Can you work these out from the model? Positions are in its coordinate system, mm. A direction names the side the tool comes from. Coordinates: 2 decimals unless noted, no trailing zeros. Loops run counter-clockwise (first coordinate to the right, second up) from the corner with the lowest first, then second, coordinate; pieces in that order, holes last. Notation, with made-up numbers: M 31.5,-39 L 59.5,-39 A27 cw 59.5,-3 Z; hole C 49.25,71 d3. An arc over 180 degrees is marked long. Answer as a JSON object with one key per item and string values. Group by question number.
Item 1: Suppose I cut it at D-D (x = 70). Write out the boundary of the cut face in (y, z).
Item 2: Suppose I cut it at C-C (z = 10). Count the separate pieces of the cut face and the enclosed holes in it, then the cut area to 3 significant figures.
Item 3: We'd pull the mould along Y, two halves only. Please class faces 1 (the flat face through (0, 27.7, 7.6)), 2 (the cylindrical face through (6.923, 48.226, 9.86)), 3 (the flat face through (27, 6, 7)): +Y half, -Y half, draft (parallel to the pull), parting line (faces both ways), or undercut.
Item 4: I'm going to push flat-ended pins straight in: pin 1 Ø10 at (y, z) = (30, 10) entering from +X; pin 2 Ø3.5 at (x, y) = (6, 50) entering from -Z; pin 3 Ø6 at (x, z) = (80.5, 10.5) entering from +Y; pin 4 Ø10 at (x, z) = (58.5, 14.5) entering from +Y. Where does each tip first touch, or does it pass through?
Item 5: If I drill on line 1 (Z direction, x = 80, y = 2.1); line 2 (X direction, y = 14, z = 17.75); line 3 (Y direction, x = 84.5, z = 1.5), over which ranges is the centre line in solid material (lowest first)?
Item 6: Which directions (+Z, -Z, +X, -X, +Y, -Y) give clear straight access to the entire face, cutting with the end or side of a thin tool? Please do faces 4 (the flat face through (12, 38, 10)), 5 (the cylindrical face through (10.028, 32.815, 4.588)), 6 (the cylindrical face through (27.185, 8.028, 4.588)).
Item 7: Suppose I cut it at A-A (x = 6). Write out the boundary of the cut face in (y, z), then the cut area to 3 significant figures.
Item 8: Suppose I cut it at B-B (y = 50). Write out the boundary of the cut face in (x, z).
```python
from build123d import *

# Parameters (mm, degrees)
SKETCH_R        = 2
PAD_DEPTH       = 20
SKETCH001_R     = 6.1
POCKET_DEPTH    = 4
SKETCH002_R     = 6.1
POCKET001_DEPTH = 4
SKETCH003_R     = 3.1
POCKET002_DEPTH = 10
SKETCH004_R     = 3.1
POCKET003_DEPTH = 10
FILLET_R        = 4
FILLET001_R     = 4
FILLET002_R     = 4
FILLET003_R     = 1
FILLET004_R     = 1


with BuildPart() as part:
    # Sketch → Pad (new body)
    with BuildSketch(Plane.XY):
        Polygon((0, 56), (12, 56), (12, 10), (100, 10), (100, 0), (0, 0), align=None)
        with Locations((6, 50)):
            Circle(SKETCH_R, mode=Mode.SUBTRACT)
        with Locations((6, 6)):
            Circle(SKETCH_R, mode=Mode.SUBTRACT)
        with Locations((90, 6)):
            Circle(SKETCH_R, mode=Mode.SUBTRACT)
        with Locations((70, 6)):
            Circle(SKETCH_R, mode=Mode.SUBTRACT)
    extrude(amount=PAD_DEPTH)

    # Sketch001 → Pocket (cut)
    with BuildSketch(Plane(origin=(0, 10, 0), x_dir=(-1, 0, 0), z_dir=(0, 1, 0))):
        with Locations((-30, 10)):
            Circle(SKETCH001_R)
        with Locations((-80, 10)):
            Circle(SKETCH001_R)
    extrude(amount=-POCKET_DEPTH, mode=Mode.SUBTRACT)

    # Sketch002 → Pocket001 (cut)
    with BuildSketch(Plane.YZ.offset(12)):
        with Locations((30, 10)):
            Circle(SKETCH002_R)
    extrude(amount=-POCKET001_DEPTH, mode=Mode.SUBTRACT)

    # Sketch003 → Pocket002 (cut)
    with BuildSketch(Plane.YZ.offset(8)):
        with Locations((30, 10)):
            Circle(SKETCH003_R)
    extrude(amount=-POCKET002_DEPTH, mode=Mode.SUBTRACT)

    # Sketch004 → Pocket003 (cut)
    with BuildSketch(Plane(origin=(0, 6, 0), x_dir=(-1, 0, 0), z_dir=(0, 1, 0))):
        with Locations((-80, 10)):
            Circle(SKETCH004_R)
        with Locations((-30, 10)):
            Circle(SKETCH004_R)
    extrude(amount=-POCKET003_DEPTH, mode=Mode.SUBTRACT)

    # Fillet
    fillet_edges = [part.edges().sort_by_distance(p)[0] for p in [
        (0, 0, 10),
    ]]
    fillet(fillet_edges, radius=FILLET_R)

    # Fillet001
    fillet001_edges = [part.edges().sort_by_distance(p)[0] for p in [
        (100, 0, 10),
    ]]
    fillet(fillet001_edges, radius=FILLET001_R)

    # Fillet002
    fillet002_edges = [part.edges().sort_by_distance(p)[0] for p in [
        (0, 56, 10),
    ]]
    fillet(fillet002_edges, radius=FILLET002_R)

    # Fillet003
    fillet003_edges = [part.edges().sort_by_distance(p)[0] for p in [
        (12, 56, 10),
    ]]
    fillet(fillet003_edges, radius=FILLET003_R)

    # Fillet004
    fillet004_edges = [part.edges().sort_by_distance(p)[0] for p in [
        (100, 10, 10),
    ]]
    fillet(fillet004_edges, radius=FILLET004_R)


solid = part.part
```
From the geometry:
{
 "1": {"outline": "M 0,0 L 4,0 L 4,20 L 0,20 Z; M 8,0 L 10,0 L 10,20 L 8,20 Z"},
 "2": {"separate pieces": "4", "enclosed holes": "4", "area": "1,220 mm2"},
 "3": {"face 1": "draft", "face 2": "undercut", "face 3": "+Y half"},
 "4": {"pin 1": "x = 8", "pin 2": "through", "pin 3": "y = 6", "pin 4": "y = 10"},
 "5": {"line 1": "0 to 6.9, 13.1 to 20", "line 2": "0 to 12", "line 3": "0 to 10"},
 "6": {"face 4": "+Z, -Z, +X, +Y", "face 5": "+X", "face 6": "+Y"},
 "7": {"outline": "M 0,0 L 4,0 L 4,20 L 0,20 Z; M 8,0 L 48,0 L 48,20 L 8,20 Z; M 52,0 L 56,0 L 56,20 L 52,20 Z; hole C 30,10 d6.2", "area": "930 mm2"},
 "8": {"outline": "M 0,0 L 4,0 L 4,20 L 0,20 Z; M 8,0 L 12,0 L 12,20 L 8,20 Z"}
}
